Work out the finished part from the listing and answer in its coordinate system (mm). A direction names the side the tool comes from. Round coordinates to 2 decimals unless told otherwise and drop trailing zeros. Order: outer loops, then holes, each group sorted by start corner. A loop starts at its lowest first (then second) coordinate and runs counter-clockwise, first axis right, second up. Notation, with made-up numbers: (13.5, -19) - (61.5, -19) arc R33 ccw to (61.5, 11) - close; hole circle Ø8 at (-6.75, -38). An arc over 180 degrees is marked (long way). Use CSV: the item, a comma, the result in double quotes.
from build123d import *

# Parameters (mm, degrees)
EXTRUDE002_DEPTH = 14.5
SKETCH003_W      = 238.445661
SKETCH003_H      = 400
EXTRUDE001_DEPTH = 14.5


with BuildPart() as extrude002:
    # Sketch001 → Extrude002 (new body, symmetric)
    with BuildSketch(Plane(origin=(0, 0, 400), x_dir=(1, 0, 0), z_dir=(0, -1, 0))):
        with BuildLine():
            add(Edge.make_bspline(
                [(23.871579, 5), (23.871579, 45), (8.871579, 45)],
                knots=[4.712389, 4.712389, 4.712389, 6.283185, 6.283185, 6.283185], degree=2, weights=[1, 0.707107, 1]))
            Line((8.871579, 45), (0, 45))
            Line((0, 45), (0, 0))
            Line((0, 0), (28.871579, 0))
            ThreePointArc((28.871579, 0), (25.336045, 1.464466), (23.871579, 5))
        make_face()
        with BuildLine():
            Line((238.445661, 3.988383), (238.445661, 0))
            Line((238.445661, 0), (170.25, 0))
            ThreePointArc((170.25, 0), (170.543307, 0.004302), (170.836361, 0.017206))
            Line((170.836361, 0.017206), (238.445661, 3.988383))
        make_face()
    extrude(amount=EXTRUDE002_DEPTH, both=True)


with BuildPart() as basin_cut:
    # Sketch003 → Extrude001 (new body, symmetric)
    with BuildSketch(Plane.XZ):
        with Locations((119.222831, 200)):
            Rectangle(SKETCH003_W, SKETCH003_H)
    extrude(amount=EXTRUDE001_DEPTH, both=True)

    # Fusion: union Extrude002
    add(extrude002.part)


solid = basin_cut.part
(1) Each of these flat-tipped pins is pushed along its axis until it touches: pin 1 (6 mm diameter, centred on x = 68, y = 3, fed in from -Z); pin 2 (8 mm diameter, centred on x = 186, y = 8.5, fed in from +Z). Where does it stop, or does it pass through?
Findings below:
pin 1,"stops at z = 0"
pin 2,"stops at z = 401.14"
(2) Find the intervals of material crossed by L1, parallel to Z at x = 117, y = -4.25; L2, parallel to X at y = 9.5, z = 412; L3, parallel to Z at x = 17.5, y = -11.75, in increasing order. Write a range as from..to.
Findings below:
L1,"z = 0..400"
L2,"x = 0..23.64"
L3,"z = 0..437.72"
(3) For faces 4 (the flat face through (238.446, 0, 197)), 5 (the flat face through (99, 0, 400)), determine the directions among +Z, -Z, +X, -X, +Y, -Y from which every point of the face is accessible in a straight line to the end or side of a thin tool.
Findings below:
face 4,"+Z, -Z, +X, +Y, -Y"
face 5,"+Z, +Y, -Y"
(4) Find section A-A (x = 36.5). Determine the outline of the cut face in (y, z).
Findings below:
outline,"(-14.5, 0) - (14.5, 0) - (14.5, 400) - (-14.5, 400) - close"
(5) The mould has two halves that part along X. Classify faces 1 (the flat face through (204.168, -0.203, 401.975)), 2 (the flat face through (4, 0, 445)), 3 (the flat face through (0, 0, 197)): released by +X, released by -X, zero draft, split by the parting line, or undercut.
Findings below:
face 1,"undercut"
face 2,"zero draft"
face 3,"released by -X"
